Design review of the part shown in the three views and the two pictorial views. Dimensions are in mm from the part's minimum x, y and z. A direction names the side the tool comes from. Coordinates: 2 decimals unless noted, no trailing zeros. Write each loop counter-clockwise with the first axis right and the second up, starting at its lowest first coordinate (ties: lowest second). Pieces come first, ordered by that corner, then holes. Notation, with made-up numbers: (57, 65) -> (99, 65) arc R33 cw to (99, 96) -> close; hole circle Ø8 at (56.5, 13.25). An arc over 180 degrees is marked (long way). Write each question's results on one line, items separated by ' | '.
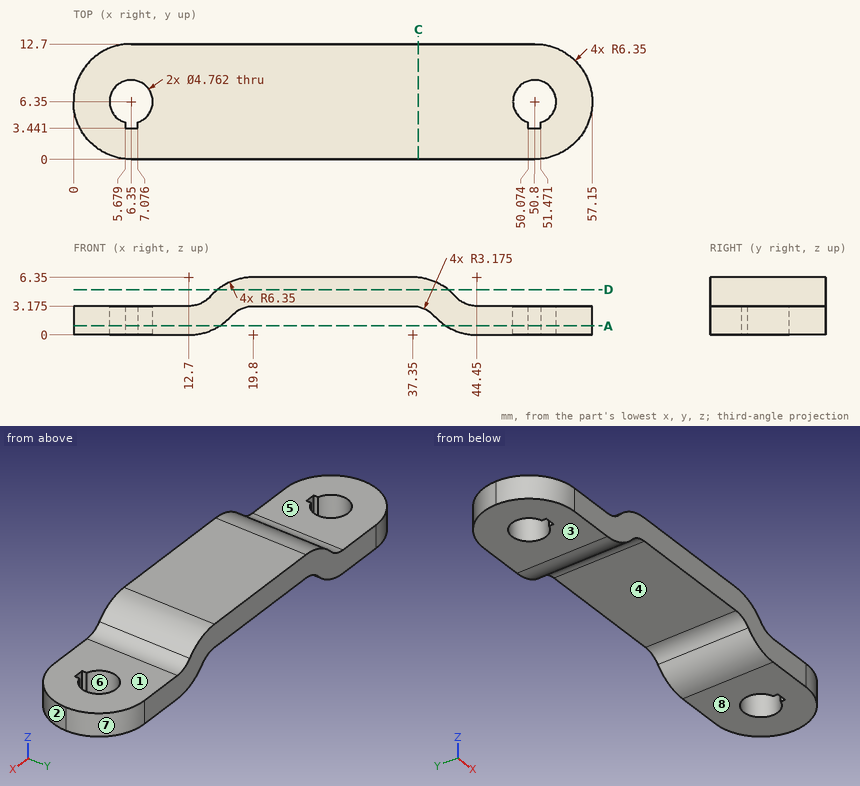
Q1. Add section A-A (z = 1). Count the separate pieces of the cut face and the enclosed holes in it, plus the area to 3 significant figures.
Solution:
separate pieces: 2 | enclosed holes: 2 | area: 338 mm²
Q2. Machinability: for the marked faces 1, 2, 3, 4 and 5, which of the approach directions +Z, -Z, +X, -X, +Y, -Y give a long, thin tool a straight path to every point of the face, cutting with its end or side? Answer none if there is none.
Solution:
face 1: +Z, +X, +Y, -Y | face 2: +Z, -Z, +X, -Y | face 3: -Z, +X, -X, +Y, -Y | face 4: -Z, +Y, -Y | face 5: +Z, -X, +Y, -Y
Q3. For line 1 (Y direction, x = 50.8, z = 1.85); line 2 (X direction, y = 6.35, z = 1.45); line 3 (X direction, y = 4.75, z = 2.5) (1 decimal), list the stretches that pass through material, from the lowest coordinate up. Write a range as from..to.
Solution:
line 1: 0..3.44, 8.73..12.7 | line 2: 0..3.97, 8.73..16.74, 40.41..48.42, 53.18..57.15 | line 3: 0.2..4.6, 8.1..17.8, 39.3..49, 52.6..56.9
Q4. Add section C-C (x = 38). Write out the cut boundary in (y, z).
Solution:
outline: (0, 3.11) -> (12.7, 3.11) -> (12.7, 6.32) -> (0, 6.32) -> close
Q5. Add section D-D (z = 5). Write out the cut boundary in (x, y) (1 decimal), plus the area to 3 significant figures.
Solution:
outline: (15.9, 0) -> (41.3, 0) -> (41.3, 12.7) -> (15.9, 12.7) -> close | area: 322 mm²
Q6. Draft analysis for pull direction Y (two halves, no side actions). For the marked faces 6, 7 and 8, state which applies: pulls with the +Y half, pulls with the -Y half, needs draft (parallel to the pull), parting line crosses it, or undercut.
Solution:
face 6: undercut | face 7: pulls with the +Y half | face 8: needs draft
Q7. Clearance check with flat-ended pins moving along their axes: P1, Ø3, axis at y = 5, z = 5.5, coming from the +X side (1 decimal); P2, Ø3, axis at y = 8.5, z = 3, coming from the +X side; P3, Ø0.7, axis at y = 3.5, z = 1.5, coming from the +X side. State where each tip first meets the part, or that it passes through.
Solution:
P1: x = 42.3 | P2: x = 57.12 | P3: x = 56.64
